Geometry: see drawing. Coordinates: mm, zero at the bounding-box minimum. Coordinates: 2 decimals unless noted, no trailing zeros. Loops run counter-clockwise (first coordinate to the right, second up) from the corner with the lowest first, then second, coordinate; pieces in that order, holes last. Notation, with made-up numbers: (69, -35.5) - (97, -35.5) arc R24 cw to (97, -10.5) - close; hole circle Ø2 at (-19, 54.5). An arc over 180 degrees is marked (long way). Use a Markdown table: item, result. Add a question column.
1. Section query A-A on z = 14.5. State how many separate pieces and enclosed holes the cut face has.
2. Ray query, L1, parallel to Z at x = 9.25, y = 0.95; L2, parallel to Z at x = 2.25, y = 0.45; L3, parallel to Y at x = 8, z = 5.5 (1 decimal). Return the intervals inside material, ascending. Write a range as [from, to].
3. Section query D-D on x = 7.5. Return the cut outline in (y, z).
4. Contact query for a flat-ended pin moving along its axis: P1, Ø4.5, axis at x = 3.16, z = 3.96, coming from the +Y side (3 decimals). Output: stop coordinate, or through.
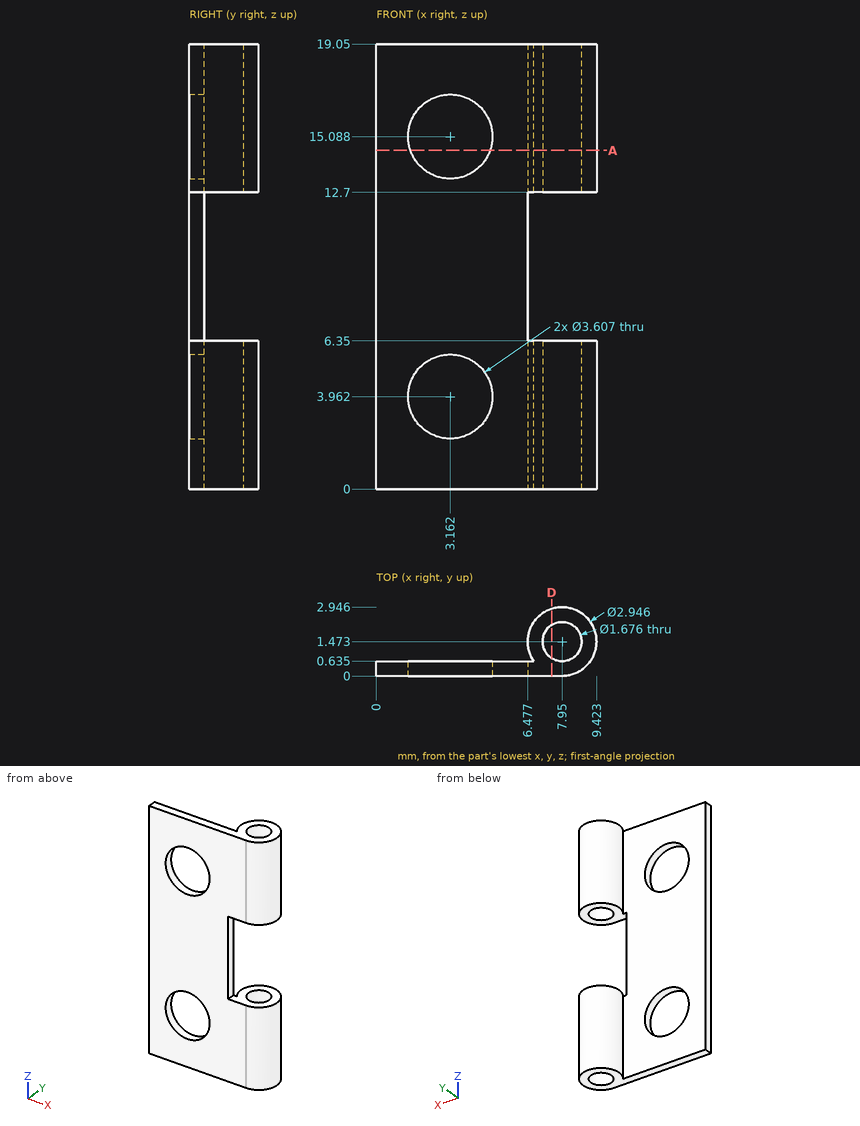
Resolved:
| question | item | result |
|---|---|---|
| 1 | separate pieces | 2 |
| 1 | enclosed holes | 1 |
| 2 | L1 | [0, 6.35], [12.7, 19.05] |
| 2 | L2 | [0, 2.41], [5.52, 13.53], [16.64, 19.05] |
| 2 | L3 | [0, 0.6], [2.3, 2.9] |
| 3 | outline | (0, 0) - (0.77, 0) - (0.77, 6.35) - (0, 6.35) - close; (0, 12.7) - (0.77, 12.7) - (0.77, 19.05) - (0, 19.05) - close; (2.18, 0) - (2.88, 0) - (2.88, 6.35) - (2.18, 6.35) - close; (2.18, 12.7) - (2.88, 12.7) - (2.88, 19.05) - (2.18, 19.05) - close |
| 4 | P1 | y = 0.635 |
